```python
from build123d import *

# Parameters (mm, degrees)
SKETCH_1_R          = 3
EXTRUDE_1_DEPTH     = 3
SKETCH_2_R          = 5
SKETCH_2_R_2        = 3
EXTRUDE_2_DEPTH     = 5
SKETCH_3_R          = 1.5
CUT_EXTRUDE_1_DEPTH = 6


with BuildPart() as part:
    # 草圖1 → 填料-伸長1 (new body)
    with BuildSketch(Plane(origin=(0, 0, 0), x_dir=(1, 0, 0), z_dir=(0, 1, 0))):
        with BuildLine():
            Line((0.333333333, 4.988876516), (30.2, 2.993325909))
            ThreePointArc((30.2, 2.993325909), (33, 0), (30.2, -2.993325909))
            Line((30.2, -2.993325909), (0.333333333, -4.988876516))
            ThreePointArc((0.333333333, -4.988876516), (-5, 0), (0.333333333, 4.988876516))
        make_face()
        Circle(SKETCH_1_R, mode=Mode.SUBTRACT)
    extrude(amount=EXTRUDE_1_DEPTH)

    # 草圖2 → 填料-伸長2 (add)
    with BuildSketch(Plane.XZ):
        Circle(SKETCH_2_R)
        Circle(SKETCH_2_R_2, mode=Mode.SUBTRACT)
    extrude(amount=EXTRUDE_2_DEPTH)

    # 草圖3 → 除料-伸長1 (cut, through all)
    with BuildSketch(Plane(origin=(0, 0, 0), x_dir=(0, 0, -1), z_dir=(1, 0, 0))):
        with Locations((0, -1)):
            Circle(SKETCH_3_R)
    extrude(amount=-CUT_EXTRUDE_1_DEPTH, mode=Mode.SUBTRACT)


solid = part.part
```
Part model, mm, in its own coordinate system. Give positions to 0.01 mm unless a question says otherwise; leave off trailing zeros. Write each loop counter-clockwise with the first axis right and the second up, starting at its lowest first coordinate (ties: lowest second). Pieces come first, ordered by that corner, then holes. Notation, with made-up numbers: M 73.5,31.5 L 107.5,31.5 A19 ccw 107.5,45.5 Z; hole C -26,13 d5. An arc over 180 degrees is marked long. Use CSV: the item, a comma, the result in double quotes.
Item 1: Drill centre lines: probe 1 along Z at (x, y) = (0, -1); probe 2 along Y at (x, z) = (13, 4); probe 3 along Z at (x, y) = (-4.25, -1). Where is each one in solid material? Low to high.
Taken from the geometry:
probe 1,"z = -5 to -3, 3 to 5"
probe 2,"y = 0 to 3"
probe 3,"z = -2.63 to -1.5, 1.5 to 2.63"
Item 2: Pin check, flat tips, straight feed: P1, Ø4, axis at x = 16.5, y = 2, coming from the -Z side; P2, Ø1, axis at x = 14, z = -3, coming from the -Y side; P3, Ø1.5, axis at y = 1.5, z = 3.5, coming from the +X side; P4, Ø5, axis at x = 0, z = 0, coming from the -Y side. Stop position of each tip, or through.
Taken from the geometry:
P1,"stops at z = -4.04"
P2,"stops at y = 0"
P3,"stops at x = 31.2"
P4,"passes through"
Item 3: Slice it at C-C on z = 2.5. Write the cut outline in (x, y).
Taken from the geometry:
outline,"M -4.33,-5 L -1.66,-5 L -1.66,3 L -4.33,3 Z; M 1.66,-5 L 4.33,-5 L 4.33,0 L 31.66,0 L 31.66,3 L 1.66,3 Z"
Item 4: Slice it at D-D on y = -3.5. Write the cut outline in (x, z), plus the area to 3 significant figures.
Taken from the geometry:
outline,"C 0,0 d10; hole C 0,0 d6"
area,"50.3 mm²"
Item 5: Slice it at A-A on x = 0. Write the cut outline in (y, z), plus the area to 3 significant figures.
Taken from the geometry:
outline,"M -5,-5 L 3,-5 L 3,-3 L -5,-3 Z; M -5,3 L 3,3 L 3,5 L -5,5 Z"
area,"32.0 mm²"
Item 6: Slice it at B-B on z = 0. Write the cut outline in (x, y).
Taken from the geometry:
outline,"M -5,-5 L -3,-5 L -3,-2.5 L -5,-2.5 Z; M -5,0.5 L -3,0.5 L -3,3 L -5,3 Z; M 3,-5 L 5,-5 L 5,0 L 33,0 L 33,3 L 3,3 Z"
Item 7: Pull direction Y, two halves, no side cores. Call faces 1 (the face through (-0.1, -5, -3.3)), 2 (the face through (-3.782, -1.575, -1.386)), 3 (the face through (33, 1, 0)): +Y half, -Y half, draft (parallel to the pull), parting line (faces both ways), or undercut.
Taken from the geometry:
face 1,"-Y half"
face 2,"undercut"
face 3,"draft"
